Check sheet for the drawn part. Datum: minimum x, y, z corner. Units: mm. Round coordinates to 2 decimals unless told otherwise and drop trailing zeros. Loops run counter-clockwise (first coordinate to the right, second up) from the corner with the lowest first, then second, coordinate; pieces in that order, holes last.
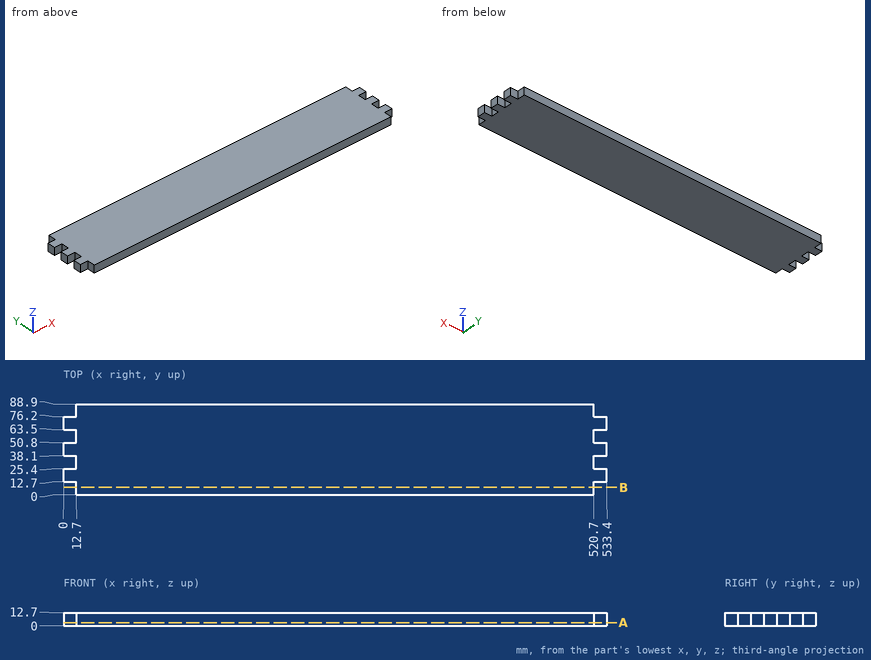
1) Sectioned sample at B-B, the plane y = 7. Record the cut outline in (x, z).
Report:
outline: (12.7, 0) - (520.7, 0) - (520.7, 12.7) - (12.7, 12.7) - close
2) Gauge pin test, flat ends, axial feed: pin 1 (6.5 mm diameter, centred on x = 5.5, z = 8.5, fed in from +Y); pin 2 (6.5 mm diameter, centred on y = 4, z = 8, fed in from +X); pin 3 (6.5 mm diameter, centred on y = 58.5, z = 9.5, fed in from -X); pin 4 (4 mm diameter, centred on x = 81, y = 67, fed in from -Z). Record the tip position at first contact, or that the pin passes through.
Report:
pin 1: stops at y = 76.2
pin 2: stops at x = 520.7
pin 3: stops at x = 12.7
pin 4: stops at z = 0
3) Scan line: line 1 along X through (y, z) = (79.5, 5.75). Record every from-to range of solid material in increasing order.
Report:
line 1: x = 12.7 to 520.7
4) Sectioned sample at A-A, the plane z = 2.75. Record the cut outline in (x, y), then the cut area to 3 significant figures.
Report:
outline: (0, 12.7) - (12.7, 12.7) - (12.7, 0) - (520.7, 0) - (520.7, 12.7) - (533.4, 12.7) - (533.4, 25.4) - (520.7, 25.4) - (520.7, 38.1) - (533.4, 38.1) - (533.4, 50.8) - (520.7, 50.8) - (520.7, 63.5) - (533.4, 63.5) - (533.4, 76.2) - (520.7, 76.2) - (520.7, 88.9) - (12.7, 88.9) - (12.7, 76.2) - (0, 76.2) - (0, 63.5) - (12.7, 63.5) - (12.7, 50.8) - (0, 50.8) - (0, 38.1) - (12.7, 38.1) - (12.7, 25.4) - (0, 25.4) - close
area: 46,100 mm2
